Geometry: final body of the model. Coordinates: model frame, mm. A direction names the side the tool comes from. Round coordinates to 2 decimals unless told otherwise and drop trailing zeros. Loops run counter-clockwise (first coordinate to the right, second up) from the corner with the lowest first, then second, coordinate; pieces in that order, holes last. Notation, with made-up numbers: M 35.25,-4 L 90.25,-4 A23 cw 90.25,34 Z; hole C 37,47 d1. An arc over 180 degrees is marked long. Answer as a JSON object with one key per item and string values.
from build123d import *

# Parameters (mm, degrees)
SKETCH1_W           = 95.5
SKETCH1_H           = 40
BOSS_EXTRUDE1_DEPTH = 100


with BuildPart() as part:
    # Sketch1 → Boss-Extrude1 (new body)
    with BuildSketch(Plane.XY):
        Polygon((-97, 0), (97, 0), (97, -180), (100, -180), (100, 89), (-100, 89), (-100, -180), (-97, -180), align=None)
        with Locations((-49.25, 23)):
            Rectangle(SKETCH1_W, SKETCH1_H, mode=Mode.SUBTRACT)
        with Locations((-49.25, 66)):
            Rectangle(SKETCH1_W, SKETCH1_H, mode=Mode.SUBTRACT)
        with Locations((49.25, 66)):
            Rectangle(SKETCH1_W, SKETCH1_H, mode=Mode.SUBTRACT)
        with Locations((49.25, 23)):
            Rectangle(SKETCH1_W, SKETCH1_H, mode=Mode.SUBTRACT)
    extrude(amount=BOSS_EXTRUDE1_DEPTH)


solid = part.part
1) Pull-direction query (Y, two-part tool) for faces 3 (the flat face through (100, -47, 49)), 4 (the flat face through (1, 89, 49)), 5 (the flat face through (-50, 46, 49)); classes: +Y half, -Y half, draft (parallel to the pull), parting line (faces both ways), or undercut.
Results:
{"face 3": "draft", "face 4": "+Y half", "face 5": "undercut"}
2) Section query D-D (y = -137.5). Return the cut outline in (x, z), and give its area (3 significant figures).
Results:
{"outline": "M -100,0 L -97,0 L -97,100 L -100,100 Z; M 97,0 L 100,0 L 100,100 L 97,100 Z", "area": "600 mm2"}
3) Ray query, line 1 (Y direction, x = 45, z = 51); line 2 (X direction, y = 41.5, z = 69.5); line 3 (X direction, y = -94, z = 44). Return the intervals inside material, ascending.
Results:
{"line 1": "0 to 3, 43 to 46, 86 to 89", "line 2": "-100 to -97, -1.5 to 1.5, 97 to 100", "line 3": "-100 to -97, 97 to 100"}
4) Section query A-A (y = 70). Return the cut outline in (x, z), and give its area (3 significant figures).
Results:
{"outline": "M -100,0 L -97,0 L -97,100 L -100,100 Z; M -1.5,0 L 1.5,0 L 1.5,100 L -1.5,100 Z; M 97,0 L 100,0 L 100,100 L 97,100 Z", "area": "900 mm2"}
5) Section query B-B (x = 14). Return the cut outline in (y, z), and give its area (3 significant figures).
Results:
{"outline": "M 0,0 L 3,0 L 3,100 L 0,100 Z; M 43,0 L 46,0 L 46,100 L 43,100 Z; M 86,0 L 89,0 L 89,100 L 86,100 Z", "area": "900 mm2"}
6) Section query C-C (z = 63). Return the cut outline in (x, y), and give its area (3 significant figures).
Results:
{"outline": "M -100,-180 L -97,-180 L -97,0 L 97,0 L 97,-180 L 100,-180 L 100,89 L -100,89 Z; hole M -97,3 L -1.5,3 L -1.5,43 L -97,43 Z; hole M -97,46 L -1.5,46 L -1.5,86 L -97,86 Z; hole M 1.5,3 L 97,3 L 97,43 L 1.5,43 Z; hole M 1.5,46 L 97,46 L 97,86 L 1.5,86 Z", "area": "3,600 mm2"}
7) Reachability of faces 1 (the flat face through (-97, -91, 49)), 2 (the flat face through (-50, 86, 49)) from +Z, -Z, +X, -X, +Y, -Y: full face, straight path, thin tool, end or side. Return the list, or none.
Results:
{"face 1": "+Z, -Z, -Y", "face 2": "+Z, -Z"}
8) Pin query (flat end, axial travel): P1, Ø10, axis at x = 29, z = 77.5, coming from the -Y side. Return the tip coordinate at first contact, or that it passes through.
Results:
{"P1": "y = 0"}
